Can you work these out from the model? Positions are in its coordinate system, mm. A direction names the side the tool comes from. Give positions to 0.01 mm unless a question says otherwise; leave off trailing zeros. Order: outer loops, then holes, each group sorted by start corner. A loop starts at its lowest first (then second) coordinate and runs counter-clockwise, first axis right, second up.
Item 1: If I drill on line 1 along Y through (x, z) = (26, 13.75); line 2 along X through (y, z) = (9, 13); line 3 along Z through (x, y) = (17.5, 10.5), over which ranges is the centre line in solid material (lowest first)?
Item 2: I want a section at A-A, the plane z = 19.75. Write out the boundary of the cut face in (x, y).
Item 3: I want a section at C-C, the plane x = 11.5. Write out the boundary of the cut face in (y, z).
Item 4: I want a section at B-B, the plane y = 26. Write out the boundary of the cut face in (x, z), then the cut area to 3 significant figures.
Item 5: I'm going to push a flat-ended pin straight in: pin 1 Ø2 at (x, y) = (9.5, 88) entering from +Z. Where does the tip first touch, or does it pass through?
Item 6: Which directions (+Z, -Z, +X, -X, +Y, -Y) give clear straight access to the entire face, cutting with the end or side of a thin tool? Please do faces 1 (the flat face through (-11.2, 123.5, 25.4)), 2 (the flat face through (-61.528, 61, 13)).
Item 7: If we mould it in two halves opening along X, with no side actions, what happens to faces 3 (the flat face through (-64.068, 61, 11)), 4 (the flat face through (-12, 0, 13)), 5 (the flat face through (-12, 62, -2.54)), 6 (the flat face through (-12, 122.988, 13))? For each: +X half, -X half, draft (parallel to the pull), parting line (faces both ways), or undercut.
```python
from build123d import *

# Parameters (mm, degrees)
F0_W     = 111.9927763939
F0_H     = 27.0903408527
F1_DEPTH = 25.4
F0_W_2   = 101.1313535273
F0_H_2   = 122.9882985353
F3_T     = 2.54


with BuildPart() as f1:
    # F0 (on Top) → F1 (new body)
    with BuildSketch(Plane.XY):
        with Locations((-55.9963881969, 277.6345461607)):
            Rectangle(F0_W, F0_H)
    extrude(amount=F1_DEPTH)


with BuildPart() as f1b:
    # F0 (on Top) → F1, piece 2 (new body)
    with BuildSketch(Plane.XY):
        with Locations((-10.9623651952, 61.4941492677)):
            Rectangle(F0_W_2, F0_H_2)
    extrude(amount=F1_DEPTH)

    # F3
    f3_openings = [f1b.faces().sort_by_distance(p)[0] for p in [
        (-10.962365, 61.494149, 25.4),
    ]]
    offset(amount=F3_T, openings=f3_openings, kind=Kind.INTERSECTION)


solid = f1b.part
```
Results list:
1. line 1: y = -2.54 to 0, 122.99 to 125.53
1. line 2: x = -64.07 to -61.53, 39.6 to 42.14
1. line 3: z = -2.54 to 0
2. outline: (-64.07, -2.54) - (42.14, -2.54) - (42.14, 125.53) - (-64.07, 125.53) - close; hole (-61.53, 0) - (39.6, 0) - (39.6, 122.99) - (-61.53, 122.99) - close
3. outline: (-2.54, -2.54) - (125.53, -2.54) - (125.53, 25.4) - (122.99, 25.4) - (122.99, 0) - (0, 0) - (0, 25.4) - (-2.54, 25.4) - close
4. outline: (-64.07, -2.54) - (42.14, -2.54) - (42.14, 25.4) - (39.6, 25.4) - (39.6, 0) - (-61.53, 0) - (-61.53, 25.4) - (-64.07, 25.4) - close
4. area: 399 mm2
5. pin 1: stops at z = 0
6. face 1: +Z, +X, -X, +Y, -Y
6. face 2: +Z
7. face 3: -X half
7. face 4: undercut
7. face 5: draft
7. face 6: undercut
